Input: part model. Units: mm. Frame: model coordinates. A direction names the side the tool comes from. Coordinates: 2 decimals unless noted, no trailing zeros.
from build123d import *

# Parameters (mm, degrees)
SKETCH_1_W          = 50.3
SKETCH_1_H          = 19
EXTRUDE_1_DEPTH     = 8
SKETCH_2_R          = 0.4
EXTRUDE_2_DEPTH     = 1.8
SKETCH_3_R          = 0.675
CUT_EXTRUDE_1_DEPTH = 0.25


with BuildPart() as part:
    # 草图1 → 凸台-拉伸1 (new body)
    with BuildSketch(Plane.XY):
        with Locations((25.15, 9.5)):
            Rectangle(SKETCH_1_W, SKETCH_1_H)
    extrude(amount=EXTRUDE_1_DEPTH)

    # 草图2 → 凸台-拉伸2 (add)
    with BuildSketch(Plane(origin=(0, 0, 0), x_dir=(-1, 0, 0), z_dir=(0, 0, -1))):
        with Locations((-31.5, 17.12)):
            Circle(SKETCH_2_R)
        with Locations((-28.96, 17.12)):
            Circle(SKETCH_2_R)
        with Locations((-26.42, 17.12)):
            Circle(SKETCH_2_R)
        with Locations((-23.88, 17.12)):
            Circle(SKETCH_2_R)
        with Locations((-21.34, 17.12)):
            Circle(SKETCH_2_R)
        with Locations((-18.8, 17.12)):
            Circle(SKETCH_2_R)
        with Locations(Location((-18.8, 1.88, 0), (0, 0, 180))):
            Circle(SKETCH_2_R)
        with Locations(Location((-21.34, 1.88, 0), (0, 0, 180))):
            Circle(SKETCH_2_R)
        with Locations(Location((-23.88, 1.88, 0), (0, 0, 180))):
            Circle(SKETCH_2_R)
        with Locations(Location((-26.42, 1.88, 0), (0, 0, 180))):
            Circle(SKETCH_2_R)
        with Locations(Location((-28.96, 1.88, 0), (0, 0, 180))):
            Circle(SKETCH_2_R)
        with Locations(Location((-31.5, 1.88, 0), (0, 0, 180))):
            Circle(SKETCH_2_R)
    extrude(amount=EXTRUDE_2_DEPTH)

    # 草图3 → 切除-拉伸1 (cut)
    # profile 1 of 8: a face of its own
    with BuildSketch(Plane.XY.offset(8)):
        with BuildLine():
            ThreePointArc((9.312943073, 3.260826899), (8.978734033, 2.64529042), (8.322675004, 2.4))
            Line((8.322675004, 2.4), (2.162726812, 2.4))
            ThreePointArc((2.162726812, 2.4), (1.408017232, 2.743940971), (1.172458743, 3.539173101))
            Line((1.172458743, 3.539173101), (2.887056927, 15.739173101))
            ThreePointArc((2.887056927, 15.739173101), (3.221265967, 16.35470958), (3.877324996, 16.6))
            Line((3.877324996, 16.6), (10.037273188, 16.6))
            ThreePointArc((10.037273188, 16.6), (10.791982768, 16.256059029), (11.027541257, 15.460826899))
            Line((11.027541257, 15.460826899), (9.312943073, 3.260826899))
        make_face()
        Polygon((3.468330618, 10.175), (8.921399509, 10.175), (9.634644245, 15.25), (4.181575354, 15.25), align=None, mode=Mode.SUBTRACT)
        Polygon((3.278600491, 8.825), (2.565355755, 3.75), (8.018424646, 3.75), (8.731669382, 8.825), align=None, mode=Mode.SUBTRACT)
    # profile 2 of 8: a face of its own
    with BuildSketch(Plane.XY.offset(8)):
        with BuildLine():
            Line((23.727541257, 15.460826899), (22.012943073, 3.260826899))
            ThreePointArc((22.012943073, 3.260826899), (21.678734033, 2.64529042), (21.022675004, 2.4))
            Line((21.022675004, 2.4), (14.862726812, 2.4))
            ThreePointArc((14.862726812, 2.4), (14.108017232, 2.743940971), (13.872458743, 3.539173101))
            Line((13.872458743, 3.539173101), (15.587056927, 15.739173101))
            ThreePointArc((15.587056927, 15.739173101), (15.921265967, 16.35470958), (16.577324996, 16.6))
            Line((16.577324996, 16.6), (22.737273188, 16.6))
            ThreePointArc((22.737273188, 16.6), (23.491982768, 16.256059029), (23.727541257, 15.460826899))
        make_face()
        Polygon((16.168330618, 10.175), (21.621399509, 10.175), (22.334644245, 15.25), (16.881575354, 15.25), align=None, mode=Mode.SUBTRACT)
        Polygon((15.265355755, 3.75), (20.718424646, 3.75), (21.431669382, 8.825), (15.978600491, 8.825), align=None, mode=Mode.SUBTRACT)
    # profile 3 of 8: a face of its own
    with BuildSketch(Plane.XY.offset(8)):
        with BuildLine():
            Line((36.427541257, 15.460826899), (34.712943073, 3.260826899))
            ThreePointArc((34.712943073, 3.260826899), (34.378734033, 2.64529042), (33.722675004, 2.4))
            Line((33.722675004, 2.4), (27.562726812, 2.4))
            ThreePointArc((27.562726812, 2.4), (26.808017232, 2.743940971), (26.572458743, 3.539173101))
            Line((26.572458743, 3.539173101), (28.287056927, 15.739173101))
            ThreePointArc((28.287056927, 15.739173101), (28.621265967, 16.35470958), (29.277324996, 16.6))
            Line((29.277324996, 16.6), (35.437273188, 16.6))
            ThreePointArc((35.437273188, 16.6), (36.191982768, 16.256059029), (36.427541257, 15.460826899))
        make_face()
        Polygon((28.868330618, 10.175), (34.321399509, 10.175), (35.034644245, 15.25), (29.581575354, 15.25), align=None, mode=Mode.SUBTRACT)
        Polygon((27.965355755, 3.75), (33.418424646, 3.75), (34.131669382, 8.825), (28.678600491, 8.825), align=None, mode=Mode.SUBTRACT)
    # profile 4 of 8: a face of its own
    with BuildSketch(Plane.XY.offset(8)):
        with BuildLine():
            Line((49.127541257, 15.460826899), (47.412943073, 3.260826899))
            ThreePointArc((47.412943073, 3.260826899), (47.078734033, 2.64529042), (46.422675004, 2.4))
            Line((46.422675004, 2.4), (40.262726812, 2.4))
            ThreePointArc((40.262726812, 2.4), (39.508017232, 2.743940971), (39.272458743, 3.539173101))
            Line((39.272458743, 3.539173101), (40.987056927, 15.739173101))
            ThreePointArc((40.987056927, 15.739173101), (41.321265967, 16.35470958), (41.977324996, 16.6))
            Line((41.977324996, 16.6), (48.137273188, 16.6))
            ThreePointArc((48.137273188, 16.6), (48.891982768, 16.256059029), (49.127541257, 15.460826899))
        make_face()
        Polygon((41.568330618, 10.175), (47.021399509, 10.175), (47.734644245, 15.25), (42.281575354, 15.25), align=None, mode=Mode.SUBTRACT)
        Polygon((40.665355755, 3.75), (46.118424646, 3.75), (46.831669382, 8.825), (41.378600491, 8.825), align=None, mode=Mode.SUBTRACT)
    # profile 5 of 8: a face of its own
    with BuildSketch(Plane.XY.offset(8)):
        with Locations((10.691961742, 3.075)):
            Circle(SKETCH_3_R)
    # profile 6 of 8: a face of its own
    with BuildSketch(Plane.XY.offset(8)):
        with Locations((23.391961742, 3.075)):
            Circle(SKETCH_3_R)
    # profile 7 of 8: a face of its own
    with BuildSketch(Plane.XY.offset(8)):
        with Locations((36.091961742, 3.075)):
            Circle(SKETCH_3_R)
    # profile 8 of 8: a face of its own
    with BuildSketch(Plane.XY.offset(8)):
        with Locations((48.791961742, 3.075)):
            Circle(SKETCH_3_R)
    extrude(amount=-CUT_EXTRUDE_1_DEPTH, mode=Mode.SUBTRACT)


solid = part.part
Item 1: Ray query, probe 1 along Z at (x, y) = (37, 15.5); probe 2 along Z at (x, y) = (46.5, 15.5). Return the intervals inside material, ascending.
Response values:
probe 1: z = 0 to 8
probe 2: z = 0 to 7.75
Item 2: Draft query along Y for faces 1 (the face through (19, 13, 8)), 2 (the face through (44, 10, 7.75)), 3 (the face through (25, 0, 4)). Return one class per face: pulls with the +Y half, pulls with the -Y half, needs draft (parallel to the pull), parting line crosses it, or undercut.
Response values:
face 1: needs draft
face 2: undercut
face 3: pulls with the -Y half
Item 3: Pin query (flat end, axial travel): pin 1 Ø3 at (x, z) = (28.5, 1.5) entering from -Y; pin 2 Ø1.2 at (x, y) = (36.09, 3.08) entering from -Z; pin 3 Ø0.7 at (x, y) = (49, 3) entering from +Z. Return the tip coordinate at first contact, or that it passes through.
Response values:
pin 1: stops at y = 0
pin 2: stops at z = 0
pin 3: stops at z = 7.75
Item 4: Access query for faces 4 (the face through (7, 13, 8)), 5 (the face through (36, 3, 7.75)). Directions: +Z, -Z, +X, -X, +Y, -Y. A direction counts if a zero-diameter tool reaches every point of the face in a straight line with its end or side. Return the directions, or none.
Response values:
face 4: +Z, +X, -X, +Y, -Y
face 5: +Z
